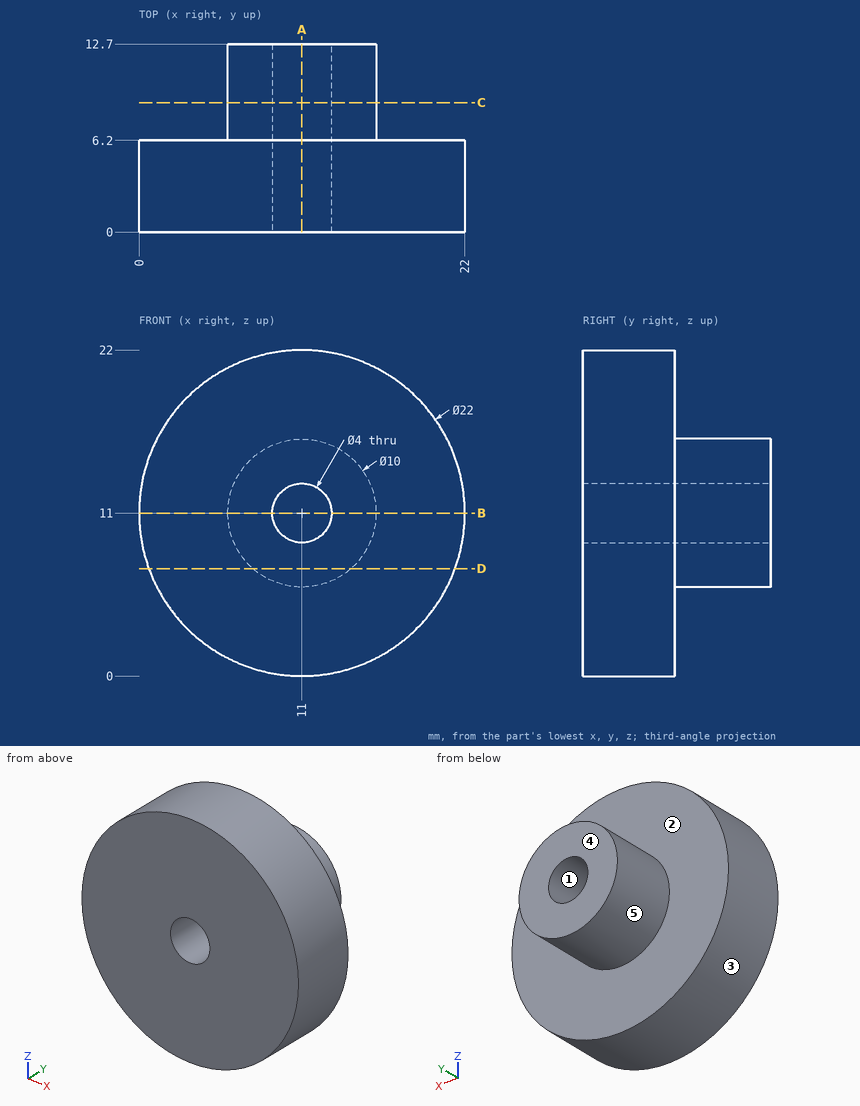
The figure shows three views and two pictorial views of one solid part (mm, origin at its lowest corner). Answer the questions. A direction names the side the tool comes from. Give positions to 0.01 mm unless a question says otherwise; leave off trailing zeros. Order: outer loops, then holes, each group sorted by start corner. A loop starts at its lowest first (then second) coordinate and runs counter-clockwise, first axis right, second up. Notation, with made-up numbers: M 76.5,0 L 107.5,0 A33 ccw 107.5,30 Z; hole C -27.5,81.5 d5. An arc over 180 degrees is marked long. Return JSON: item names as keys, results as strings.
1) Section B-B, the plane z = 11 is taken. Write down the section's boundary in (x, y), plus the area to 3 significant figures.
Resolved:
{"outline": "M 0,0 L 9,0 L 9,12.7 L 6,12.7 L 6,6.2 L 0,6.2 Z; M 13,0 L 22,0 L 22,6.2 L 16,6.2 L 16,12.7 L 13,12.7 Z", "area": "151 mm^2"}
2) For a pull along X with two mould halves and no side action, classify the marked faces 1, 2 and 3 as +X half, -X half, draft (parallel to the pull), parting line (faces both ways), or undercut.
Resolved:
{"face 1": "undercut", "face 2": "draft", "face 3": "parting line"}
3) A tool of negligible diameter and unlimited length cuts with its end or side. For the marked faces 4 and 5, from which of +Z, -Z, +X, -X, +Y, -Y can it reach the whole face along a straight path? Write none if from no direction.
Resolved:
{"face 4": "+Z, -Z, +X, -X, +Y", "face 5": "+Y"}
4) Section C-C, the plane y = 8.75 is taken. Write down the section's boundary in (x, z).
Resolved:
{"outline": "C 11,11 d10; hole C 11,11 d4"}
5) Each of these flat-tipped pins is pushed along its axis until it touches: pin 1 (1 mm diameter, centred on y = 3.5, z = 19.5, fed in from -X); pin 2 (11 mm diameter, centred on x = 11.5, z = 6, fed in from +Y); pin 3 (6 mm diameter, centred on x = 4.5, y = 4.5, fed in from +Z); pin 4 (1.5 mm diameter, centred on x = 4.5, y = 6.5, fed in from -Z). Where does it stop, or does it pass through?
Resolved:
{"pin 1": "x = 3.45", "pin 2": "y = 12.7", "pin 3": "z = 21.43", "pin 4": "z = 1.66"}
6) Section A-A, the plane x = 11 is taken. Write down the section's boundary in (y, z).
Resolved:
{"outline": "M 0,0 L 6.2,0 L 6.2,6 L 12.7,6 L 12.7,9 L 0,9 Z; M 0,13 L 12.7,13 L 12.7,16 L 6.2,16 L 6.2,22 L 0,22 Z"}
7) Section D-D, the plane z = 7.25 is taken. Write down the section's boundary in (x, y).
Resolved:
{"outline": "M 0.66,0 L 21.34,0 L 21.34,6.2 L 14.31,6.2 L 14.31,12.7 L 7.69,12.7 L 7.69,6.2 L 0.66,6.2 Z"}
8) Straight lines are drawn through the part: line 1 along Z through (x, y) = (11, 5); line 2 along Z through (x, y) = (11, 8); line 3 along Y through (x, z) = (7.75, 2). For each, find the intervals that lie inside material, in ascending order. Write a range as [from, to].
Resolved:
{"line 1": "[0, 9], [13, 22]", "line 2": "[6, 9], [13, 16]", "line 3": "[0, 6.2]"}
